```python
from build123d import *

# Parameters (mm, degrees)
F0_W     = 76.2
F0_H     = 9.1570811439
F1_DEPTH = 50.8
F3_DEPTH = 50.8
F5_D     = 25.4


with BuildPart() as f1:
    # F0 (on Front) → F1 (new body)
    with BuildSketch(Plane.XZ):
        with Locations((7.8489261553, 4.578540572)):
            Rectangle(F0_W, F0_H)
    extrude(amount=F1_DEPTH)

    # F2 (on face) → F3 (join)
    with BuildSketch(Plane.XZ.offset(50.8)):
        with BuildLine():
            Line((-17.5510738447, 9.1570811439), (33.2489261553, 9.1570811439))
            ThreePointArc((33.2489261553, 9.1570811439), (7.8489261553, 34.5570811439), (-17.5510738447, 9.1570811439))
        make_face()
    extrude(amount=-F3_DEPTH)

    # F5 (through all)
    with Locations(Plane.XZ.offset(50.8)):
        with Locations((7.8489261553, 17.78)):
            Hole(F5_D / 2)


solid = f1.part
```
Here's how the part is built. I have some questions about the finished solid (model axes, mm). A direction names the side the tool comes from. Coordinates: 2 decimals unless noted, no trailing zeros. Loops run counter-clockwise (first coordinate to the right, second up) from the corner with the lowest first, then second, coordinate; pieces in that order, holes last. Notation, with made-up numbers: (84.5, -28) -> (102.5, -28) arc R11 cw to (102.5, -15) -> close; hole circle Ø10 at (45, -17). An arc over 180 degrees is marked (long way). Return JSON: item names as keys, results as strings.
1) If we section it at D-D, the plane x = -21: Write out the boundary of the cut face in (y, z), then the cut area to 3 significant figures.
Results below:
{"outline": "(-50.8, 0) -> (0, 0) -> (0, 9.16) -> (-50.8, 9.16) -> close", "area": "465 mm²"}
2) Will these pins go through, and if not, where does the flat tip stop? pin 1 (5 mm diameter, centred on y = -30, z = 21.5, fed in from -X); pin 2 (3 mm diameter, centred on y = -39, z = 17, fed in from +X); pin 3 (1 mm diameter, centred on y = -41.5, z = 15, fed in from +X); pin 4 (3 mm diameter, centred on y = -31, z = 9.5, fed in from -X).
Results below:
{"pin 1": "x = -15.57", "pin 2": "x = 32.44", "pin 3": "x = 32.68", "pin 4": "x = -30.25"}
3) For faces 5 (the face through (40, -25, 9.157)), 6 (the face through (-24, -25, 9.157)), 7 (the face through (-30.251, -25, 5)), which set-ups out of +Z, -Z, +X, -X, +Y, -Y let a thin tool reach every point of the face, with its end or its side?
Results below:
{"face 5": "+Z, +X, +Y, -Y", "face 6": "+Z, -X, +Y, -Y", "face 7": "+Z, -Z, -X, +Y, -Y"}
4) Thinking about a two-plate mould opening in X: for faces 1 (the face through (8.41, -25.76, 34.55)), 2 (the face through (16, 0, 6)), 3 (the face through (17.927, -25.044, 10.052)), 4 (the face through (45.949, -25, 5)), which applies, +X half, -X half, draft (parallel to the pull), parting line (faces both ways), or undercut?
Results below:
{"face 1": "parting line", "face 2": "draft", "face 3": "undercut", "face 4": "+X half"}
5) If we section it at C-C, the plane x = 13.5: Write out the boundary of the cut face in (y, z).
Results below:
{"outline": "(-50.8, 0) -> (0, 0) -> (0, 6.41) -> (-50.8, 6.41) -> close; (-50.8, 29.15) -> (0, 29.15) -> (0, 33.92) -> (-50.8, 33.92) -> close"}
6) I need wall thicknesses on line 1 (Z direction, x = 7.5, y = -43.5); line 2 (Z direction, x = 12.5, y = -13); line 3 (Z direction, x = -24.5, y = -42.5). Which ranges of each line are inside material? Lowest first, please. Write a range as from..to.
Results below:
{"line 1": "0..5.08, 30.48..34.55", "line 2": "0..5.96, 29.6..34.13", "line 3": "0..9.16"}
7) If we section it at A-A, the plane y = -23.5: Write out the boundary of the cut face in (x, z).
Results below:
{"outline": "(-30.25, 0) -> (45.95, 0) -> (45.95, 9.16) -> (33.25, 9.16) arc R25.4 ccw to (-17.55, 9.16) -> (-30.25, 9.16) -> close; hole circle Ø25.4 at (7.85, 17.78)"}
8) If we section it at B-B, the plane z = 17.78: Write out the boundary of the cut face in (x, y).
Results below:
{"outline": "(-16.04, -50.8) -> (-4.85, -50.8) -> (-4.85, 0) -> (-16.04, 0) -> close; (20.55, -50.8) -> (31.74, -50.8) -> (31.74, 0) -> (20.55, 0) -> close"}
